Here's how the part is built. I have some questions about the finished solid (model axes, mm). Face numbers are marked on the shaded views. A direction names the side the tool comes from. Give positions to 0.01 mm unless a question says otherwise; leave off trailing zeros. Loops run counter-clockwise (first coordinate to the right, second up) from the corner with the lowest first, then second, coordinate; pieces in that order, holes last. Notation, with made-up numbers: (16.5, -8) -> (65.5, -8) arc R9 ccw to (65.5, -1) -> close; hole circle Ø5 at (79.5, -12.75). An arc over 180 degrees is marked (long way). Answer in a Markdown table with one row per item. Add a question column.
Item 1: For P1, Ø2.5, axis at y = 23.5, z = 20.5, coming from the -X side; P2, Ø0.5, axis at x = 22, z = 18, coming from the -Y side; P3, Ø1.6, axis at y = -23, z = 28.5, coming from the +X side; P4, Ø1, axis at x = 9.5, z = 12, coming from the -Y side, each with a flat end and sliding along its axis, tell me the tip position at first contact or that it passes through.
Item 2: Which directions (+Z, -Z, +X, -X, +Y, -Y) give clear straight access to the entire face, cutting with the end or side of a thin tool? Please do the marked faces 1 and 2.
Item 3: If we section it at B-B (x = -12): Write out the boundary of the cut face in (y, z) (3 decimals).
Item 4: If we section it at D-D (x = 19.5): Write out the boundary of the cut face in (y, z).
Item 5: If I drill on line 1 (Z direction, x = 18, y = -1.5); line 2 (X direction, y = 7, z = 14.5) (3 decimals); line 3 (X direction, y = 23.5, z = 17) (3 decimals), over which ranges is the centre line in solid material (lowest first)?
Item 6: We'd pull the mould along Z, two halves only. Please class the marked faces 3, 4, 5 and 6: released by +Z, released by -Z, zero draft, split by the parting line, or undercut.
Item 7: If we section it at C-C (y = -10): Write out the boundary of the cut face in (x, z) (3 decimals), then the cut area to 3 significant figures.
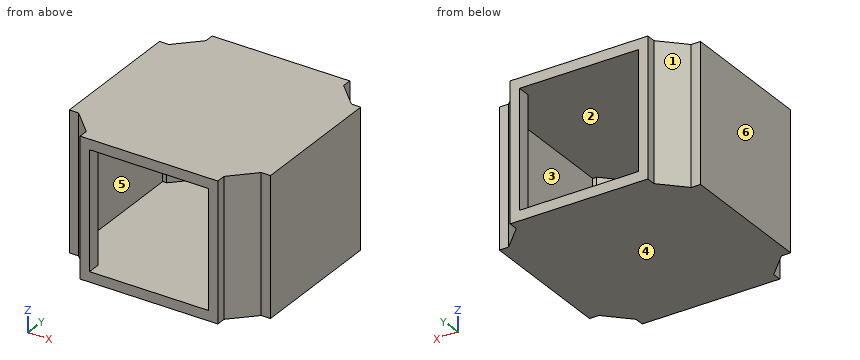
Autodesk Inventor part; units mm, degrees
ref_plane "Work Plane1" through (-24.9, -24.9, 7.7) normal (0, 0, 1) x (1, 0, 0)
ref_plane "YZ Plane" through (0, 0, 0) normal (1, 0, 0) x (0, 1, 0)
ref_plane "XZ Plane" through (0, 0, 0) normal (0, 1, 0) x (-1, 0, 0)
sketch "Sketch1" plane through (0, 0, 0) normal (0, 0, 1) x (1, 0, 0)
  circle A0 centre (-10, 20.9) radius 1.875
  circle A1 centre (-10, -20.9) radius 1.875
  circle A2 centre (10, 20.9) radius 1.875
  circle A3 centre (10, -20.9) radius 1.875
  circle A4 centre (20.8, -14.4) radius 2.075
  circle A5 centre (20.8, 14.4) radius 2.075
  circle A6 centre (-20.8, 14.4) radius 2.075
  circle A7 centre (-20.8, -14.4) radius 2.075
  line L0 (16.9, -16.9) -> (-16.9, -16.9)
  line L1 (-16.9, -16.9) -> (-16.9, 16.9)
  line L2 (-16.9, 16.9) -> (16.9, 16.9)
  line L3 (16.9, 16.9) -> (16.9, -16.9)
  line L4 (-17.05, 24.9) -> (-17.05, 22.55)
  line L5 (-17.05, 22.55) -> (-22.55, 17.05)
  line L6 (-22.55, 17.05) -> (-24.9, 17.05)
  line L7 (-24.9, 17.05) -> (-24.9, -17.05)
  line L8 (-24.9, -17.05) -> (-22.55, -17.05)
  line L9 (-22.55, -17.05) -> (-17.05, -22.55)
  line L10 (-17.05, -22.55) -> (-17.05, -24.9)
  line L11 (-17.05, -24.9) -> (17.05, -24.9)
  line L12 (17.05, -24.9) -> (17.05, -22.55)
  line L13 (17.05, -22.55) -> (22.55, -17.05)
  line L14 (22.55, -17.05) -> (24.9, -17.05)
  line L15 (24.9, -17.05) -> (24.9, 17.05)
  line L16 (24.9, 17.05) -> (22.55, 17.05)
  line L17 (22.55, 17.05) -> (17.05, 22.55)
  line L18 (17.05, 22.55) -> (17.05, 24.9)
  line L19 (17.05, 24.9) -> (-17.05, 24.9)
  line L20 (24.825, 16.975) -> (24.825, -16.975)
  line L21 (24.825, -16.975) -> (22.5189, -16.975)
  line L22 (22.5189, -16.975) -> (16.975, -22.5189)
  line L23 (16.975, -22.5189) -> (16.975, -24.825)
  line L24 (16.975, -24.825) -> (-16.975, -24.825)
  line L25 (-16.975, -24.825) -> (-16.975, -22.5189)
  line L26 (-16.975, -22.5189) -> (-22.5189, -16.975)
  line L27 (-22.5189, -16.975) -> (-24.825, -16.975)
  line L28 (-24.825, -16.975) -> (-24.825, 16.975)
  line L29 (-24.825, 16.975) -> (-22.5189, 16.975)
  line L30 (-22.5189, 16.975) -> (-16.975, 22.5189)
  line L31 (-16.975, 22.5189) -> (-16.975, 24.825)
  line L32 (-16.975, 24.825) -> (16.975, 24.825)
  line L33 (16.975, 24.825) -> (16.975, 22.5189)
  line L34 (16.975, 22.5189) -> (22.5189, 16.975)
  line L35 (22.5189, 16.975) -> (24.825, 16.975)
  point P0 (0, 0)
  dimension "d0" = 0.075
ref_plane "Work Plane1" through (-24.9, -24.9, 7.7) normal (0, 0, 1) x (1, 0, 0)
extrude "Extrusion1" add sketch "Sketch1" along normal blind 2.5 from surface at 7.7 contours A0 | A1 | A2 | A3 | A4 | A5 | A6 | A7 | L0 L1 L2 L3 | L20 L21 L22 L23 L24 L25 L26 L27 L28 L29 L30 L31 L32 L33 L34 L35
sketch "Sketch2" plane through (0, 0, 0) normal (0, 0, 1) x (1, 0, 0)
  line L0 (22.5189, 16.975) -> (24.825, 16.975)
  line L1 (16.975, 22.5189) -> (22.5189, 16.975)
  line L2 (16.975, 24.825) -> (16.975, 22.5189)
  line L3 (-16.975, 24.825) -> (16.975, 24.825)
  line L4 (-16.975, 22.5189) -> (-16.975, 24.825)
  line L5 (-22.5189, 16.975) -> (-16.975, 22.5189)
  line L6 (-24.825, 16.975) -> (-22.5189, 16.975)
  line L7 (-24.825, -16.975) -> (-24.825, 16.975)
  line L8 (-22.5189, -16.975) -> (-24.825, -16.975)
  line L9 (-16.975, -22.5189) -> (-22.5189, -16.975)
  line L10 (-16.975, -24.825) -> (-16.975, -22.5189)
  line L11 (16.975, -24.825) -> (-16.975, -24.825)
  line L12 (16.975, -22.5189) -> (16.975, -24.825)
  line L13 (22.5189, -16.975) -> (16.975, -22.5189)
  line L14 (24.825, -16.975) -> (22.5189, -16.975)
  line L15 (24.825, 16.975) -> (24.825, -16.975)
  line L16 (24.825, -16.975) -> (22.5189, -16.975)
  line L17 (22.5189, -16.975) -> (22.5189, 16.975)
  line L18 (22.5189, 16.975) -> (24.825, 16.975)
  line L19 (24.825, 16.975) -> (24.825, -16.975)
  line L20 (-22.5189, 16.975) -> (-24.825, 16.975)
  line L21 (-24.825, 16.975) -> (-24.825, -16.975)
  line L22 (-24.825, -16.975) -> (-22.5189, -16.975)
  line L23 (-22.5189, -16.975) -> (-22.5189, 16.975)
  line L24 (22.525, -14.675) -> (21.5662, -14.675)
  line L25 (21.5662, -14.675) -> (14.675, -21.5662)
  line L26 (14.675, -21.5662) -> (14.675, -22.525)
  line L27 (14.675, -22.525) -> (-14.675, -22.525)
  line L28 (-14.675, -22.525) -> (-14.675, -21.5662)
  line L29 (-14.675, -21.5662) -> (-21.5662, -14.675)
  line L30 (-21.5662, -14.675) -> (-22.525, -14.675)
  line L31 (-22.525, -14.675) -> (-22.525, 14.675)
  line L32 (-22.525, 14.675) -> (-21.5662, 14.675)
  line L33 (-21.5662, 14.675) -> (-14.675, 21.5662)
  line L34 (-14.675, 21.5662) -> (-14.675, 22.525)
  line L35 (-14.675, 22.525) -> (14.675, 22.525)
  line L36 (14.675, 22.525) -> (14.675, 21.5662)
  line L37 (14.675, 21.5662) -> (21.5662, 14.675)
  line L38 (21.5662, 14.675) -> (22.525, 14.675)
  line L39 (22.525, 14.675) -> (22.525, -14.675)
  line L40 (14.675, 22.525) -> (14.675, 24.825)
  line L41 (-14.675, 22.525) -> (-14.675, 24.825)
  line L42 (-14.675, -22.525) -> (-14.675, -24.825)
  line L43 (14.675, -22.525) -> (14.675, -24.825)
  point P0 (0, 0)
  dimension "d3" = 2.3
extrude "Extrusion2" add sketch "Sketch2" along normal blind 31.5 from surface at 10.2 contours L17 L38 L37 L36 L40 L3 L2 L1 | L0 L15 L14 L17 L24 L39 L38 | L17 L13 L12 L11 L43 L26 L25 L24 | L41 L34 L33 L32 L23 L5 L4 L3 | L42 L11 L10 L9 L23 L30 L29 L28 | L23 L32 L31 L30 L8 L7 L6
extrude "Extrusion3" add sketch "Sketch2" against normal blind 2.5 from surface at 41.7
properties part number "Tunnel Horizontal"
Recorded:
| question | item | result |
|---|---|---|
| 1 | P1 | stops at x = -17.24 |
| 1 | P2 | stops at y = -17.74 |
| 1 | P3 | stops at x = 17.29 |
| 1 | P4 | passes through |
| 2 | face 1 | +Z, -Z, -X, +Y |
| 2 | face 2 | none |
| 3 | outline | (-24.825, 7.7) -> (24.825, 7.7) -> (24.825, 10.2) -> (-24.825, 10.2) -> close; (-24.825, 39.2) -> (24.825, 39.2) -> (24.825, 41.7) -> (-24.825, 41.7) -> close |
| 4 | outline | (-19.99, 7.7) -> (19.99, 7.7) -> (19.99, 41.7) -> (-19.99, 41.7) -> close; hole (-16.74, 10.2) -> (16.74, 10.2) -> (16.74, 39.2) -> (-16.74, 39.2) -> close |
| 5 | line 1 | z = 7.7 to 10.2, 39.2 to 41.7 |
| 5 | line 2 | x = -24.825 to -22.525, 22.525 to 24.825 |
| 5 | line 3 | x = -16.975 to -14.675, 14.675 to 16.975 |
| 6 | face 3 | undercut |
| 6 | face 4 | released by -Z |
| 6 | face 5 | undercut |
| 6 | face 6 | zero draft |
| 7 | outline | (-24.825, 7.7) -> (24.825, 7.7) -> (24.825, 41.7) -> (-24.825, 41.7) -> close; hole (-22.525, 10.2) -> (22.525, 10.2) -> (22.525, 39.2) -> (-22.525, 39.2) -> close |
| 7 | area | 382 mm^2 |
